The model under review builds one solid part; all positions refer to its coordinate system, in mm. A direction names the side the tool comes from. Give positions to 0.01 mm unless a question says otherwise; leave off trailing zeros. Write each loop counter-clockwise with the first axis right and the second up, starting at its lowest first coordinate (ties: lowest second). Pieces come first, ordered by that corner, then holes.
Autodesk Inventor part; units mm, degrees
ref_plane "YZ Plane" through (0, 0, 0) normal (1, 0, 0) x (0, 1, 0)
ref_plane "XZ Plane" through (0, 0, 0) normal (0, 1, 0) x (-1, 0, 0)
ref_plane "XY Plane" through (0, 0, 0) normal (0, 0, 1) x (1, 0, 0)
sketch "스케치1" plane through (0, 0, 0) normal (0, 0, 1) x (1, 0, 0)
  line L0 (0, 0) -> (0, 32.9047)
  line L1 (0, 0) -> (28.5, 0)
  line L2 (28.5, 0) -> (28.5, 2.8)
  line L3 (28.5, 2.8) -> (26.075, 2.8)
  line L4 (26.075, 2.8) -> (26.075, 4.05)
  line L5 (26.075, 4.05) -> (0, 4.05)
  line L6 (28.5, 2.8) -> (28.5, 1)
  line L7 (28.5, 1) -> (27.9, 1)
  line L8 (27.9, 1) -> (27.9, 0)
  line L9 (27.9, 0) -> (26.3, 0)
  line L10 (26.3, 0) -> (26.3, 1.75)
  line L11 (-6.25, 2) -> (6.25, 2)
  arc A0 (-6.25, 2) -> (6.25, 2) centre (0, 21.0312) ccw
  line L12 (0, 1) -> (0, 2)
  arc A1 (6.25, 2) -> (26.3, 1.75) centre (18.9509, 216.4804) ccw
  line L13 (26.3, 1.75) -> (26.3, 1.95)
  line L14 (26.3, 1.95) -> (0, 2.4617)
  line L15 (26.3, 1.95) -> (26.3, 2.4617)
  line L16 (26.3, 2.4617) -> (25.7694, 2.4617)
  line L17 (25.7694, 2.4617) -> (25.7694, 3.656)
  line L18 (25.7694, 3.656) -> (0, 3.656)
  point P0 (0, 1)
  dimension "d1" = 28.5
  dimension "d2" = 2.8
  dimension "d3" = 26.075
  dimension "d4" = 1.25
  dimension "d5" = 1.8
  dimension "d6" = 0.6
  dimension "d7" = 1.6
  dimension "d8" = 1.75
  dimension "d9" = 12.5
  dimension "d10" = 0.8
  dimension "d11" = 1
  dimension "d19" = 0.2
revolve "회전1" add sketch "스케치1" angle 360 about axis through (0, 0, 0) along (0, 1, 0) picked at (3.4853, 1.8155) contours L0 L11 A0 | L10 L13 L15 L16 L17 L18 L0 L5 L4 L3 L2 L7 L8 L1 | L0 L14 L13 A1 L11
sketch "스케치2" plane through (0, 4.05, 0) normal (0, 1, 0) x (1, 0, 0)
  circle A0 centre (0, 0) radius 15.275
  dimension "d13" = 30.55
extrude "돌출1" add sketch "스케치2" along normal blind 1.2
sketch "스케치3" plane through (0, 5.25, 0) normal (0, 1, 0) x (1, 0, 0)
  circle A0 centre (0, 0) radius 9
  dimension "d16" = 18
extrude "돌출2" add sketch "스케치3" along normal blind 2.5
sketch "스케치4" plane through (0, 4.05, 0) normal (0, 1, 0) x (1, 0, 0)
  point P0 (0, 0)
sketch "스케치5" plane through (0, 4.05, 0) normal (0, 1, 0) x (1, 0, 0)
  circle A0 centre (0, 19.25) radius 2.75
  line L0 (0, 19.25) -> (0, 0)
  dimension "d20" = 5.5
  dimension "d21" = 19.25
extrude "돌출3" cut sketch "스케치5" against normal blind 0.5
pattern_circular "원형 패턴1" count 12 over 360 about axis through (0, 4.05, 0) along (0, 1, 0) of "돌출3"
sketch "스케치6" plane through (0, 4.05, 0) normal (0, 1, 0) x (1, 0, 0)
  circle A0 centre (0, -19.25) radius 2.75
  point P0 (0, 0)
extrude "돌출4" add sketch "스케치6" against normal blind 0.5
properties part number "speaker"
1) Insertion check: pin 1 (5 mm diameter, centred on x = -19.25, z = 0, fed in from -Y); pin 2 (2 mm diameter, centred on x = 5.5, y = 3.5, fed in from -Z); pin 3 (5 mm diameter, centred on x = 0, z = -14.5, fed in from +Y). Each pin has a flat end and moves straight along its axis. Give the tip position at first contact, or say it passes through.
2) Consider section A-A, the plane y = 6. Give the boundary of the cut face in (x, z).
3) To check wall thickness, follow probe 1 along X at (y, z) = (3.9, 0) (3 decimals); probe 2 along Z at (x, y) = (0, 2.85) (3 decimals); probe 3 along Z at (x, y) = (0.5, 3.75). State the ranges of each line that lie inside material, in increasing order.
4) The part is to be moulded in two halves that separate along Z. For faces 1 (the flat face through (-19, 0, -19)), 2 (the cylindrical face through (17.03, 3.86, -6.9)), 3 (the cylindrical face through (-5.653, 3.434, 25.455)), say which applies: +Z half, -Z half, draft (parallel to the pull), parting line (faces both ways), or undercut.
5) Tool access review of faces 4 (the cylindrical face through (-26.275, 0.887, -1.156)), 5 (the cylindrical face through (-1.172, 6.482, 8.923)), 6 (the cylindrical face through (-26.275, 2.209, -1.156)): name each direction out of +Z, -Z, +X, -X, +Y, -Y from which nothing blocks a thin tool from reaching the whole face with its end or side.
Answer block:
1. pin 1: stops at y = 1.62
1. pin 2: stops at z = -28.1
1. pin 3: stops at y = 5.25
2. outline: circle Ø18 at (0, 0)
3. probe 1: x = -26.075 to -22, -16.5 to 16.5, 22 to 26.075
3. probe 2: z = -26.075 to -25.769, 25.769 to 26.075
3. probe 3: z = -26.07 to -21.95, -16.55 to 26.07
4. face 1: draft
4. face 2: undercut
4. face 3: parting line
5. face 4: -Y
5. face 5: +Y
5. face 6: none
